from build123d import *

# Parameters (mm, degrees)
SKETCH1_W           = 40
SKETCH1_H           = 30
BOSS_EXTRUDE1_DEPTH = 5
SKETCH2_R           = 1.5
BOSS_EXTRUDE2_DEPTH = 40
SKETCH4_R           = 1.5
BOSS_EXTRUDE4_DEPTH = 5


with BuildPart() as part:
    # Sketch1 → Boss-Extrude1 (new body)
    with BuildSketch(Plane(origin=(0, 0, 0), x_dir=(1, 0, 0), z_dir=(0, 1, 0))):
        with Locations((20, -15)):
            Rectangle(SKETCH1_W, SKETCH1_H)
    extrude(amount=BOSS_EXTRUDE1_DEPTH)

    # Sketch2 → Boss-Extrude2 (add)
    with BuildSketch(Plane.ZY):
        with BuildLine():
            ThreePointArc((8.106694093, 9.054477386), (4.053347046, 13.107824432), (0, 9.054477386))
            Line((0, 9.054477386), (0, 5))
            Line((0, 5), (12.116930909, 5))
            ThreePointArc((12.116930909, 5), (9.279911424, 6.188818307), (8.106633421, 9.032299844))
            ThreePointArc((8.106633421, 9.032299844), (8.106678925, 9.043388574), (8.106694093, 9.054477386))
        make_face()
        with Locations((4.053347046, 9.054477386)):
            Circle(SKETCH2_R, mode=Mode.SUBTRACT)
    extrude(amount=-BOSS_EXTRUDE2_DEPTH)

    # Sketch4 → Boss-Extrude4 (add)
    with BuildSketch(Plane.ZY):
        with BuildLine():
            Line((30, 5), (28.232674565, 29.357717289))
            ThreePointArc((28.232674565, 29.357717289), (24.143809842, 33.243814974), (19.891005174, 29.537843793))
            Line((19.891005174, 29.537843793), (17.041462837, 5))
            Line((17.041462837, 5), (30, 5))
        make_face()
        with Locations((24.053347046, 29.054477386)):
            Circle(SKETCH4_R, mode=Mode.SUBTRACT)
    extrude(amount=-BOSS_EXTRUDE4_DEPTH)


solid = part.part
Model file for the job. Use its own axes, mm. A direction names the side the tool comes from. Coordinates: 2 decimals unless noted, no trailing zeros. Order: outer loops, then holes, each group sorted by start corner. A loop starts at its lowest first (then second) coordinate and runs counter-clockwise, first axis right, second up. Notation, with made-up numbers: (39, 69.25) -> (74, 69.25) arc R27 ccw to (74, 106.25) -> close; hole circle Ø10 at (63.5, 80.25). An arc over 180 degrees is marked (long way). Return JSON: item names as keys, results as strings. Group by question number.
Item 1: Tool access for faces 4 (the flat face through (0, 13, 21)), 5 (the flat face through (5, 16, 23)), 6 (the flat face through (2.465, 17.441, 18.486)): list every direction of +Z, -Z, +X, -X, +Y, -Y with a clear straight run to the whole face (end or side of a thin tool).
Item 2: Saw through at C-C on y = 8.5. Write the cut outline in (x, z), then the cut area to 3 significant figures.
Item 3: Flat gauge pins, fed straight in: P1, Ø2, axis at x = 22, z = 17.5, coming from the +Y side; P2, Ø3.5, axis at y = 29.05, z = 24.05, coming from the +X side; P3, Ø8, axis at x = 9.5, z = 10.5, coming from the +Y side. Where does each tip first touch, or does it go through?
Item 4: Saw through at B-B on z = 3.75. Write the cut outline in (x, y), then the cut area to 3 significant figures.
Item 5: Wall check: line 1 along X through (y, z) = (14, 25.75); line 2 along Y through (x, z) = (15.5, 5.25). Give the ranges that are in metal, low to high. Write a range as [from, to].
Item 6: Saw through at D-D on x = 4. State how many separate pieces and enclosed holes the cut face has, then the cut area to 3 significant figures.
Item 7: Pull direction Z, two halves, no side cores. Call faces 1 (the flat face through (20, 0, 15)), 2 (the cylindrical face through (2.46, 33.24, 24.23)), 3 (the cylindrical face through (19.72, 10.32, 4.86)): pulls with the +Z half, pulls with the -Z half, needs draft (parallel to the pull), parting line crosses it, or undercut.
Values found:
{
 "1": {"face 4": "+Z, -Z, -X, +Y, -Y", "face 5": "+Z, +X, +Y", "face 6": "+X, -X, +Y"},
 "2": {"outline": "(0, 0) -> (40, 0) -> (40, 2.66) -> (0, 2.66) -> close; (0, 5.45) -> (40, 5.45) -> (40, 8.14) -> (0, 8.14) -> close; (0, 17.45) -> (5, 17.45) -> (5, 29.75) -> (0, 29.75) -> close", "area": "276 mm2"},
 "3": {"P1": "stops at y = 5", "P2": "stops at x = 5", "P3": "stops at y = 12.29"},
 "4": {"outline": "(0, 0) -> (40, 0) -> (40, 7.59) -> (0, 7.59) -> close; (0, 10.52) -> (40, 10.52) -> (40, 13.1) -> (0, 13.1) -> close", "area": "406 mm2"},
 "5": {"line 1": "x = [0, 5]", "line 2": "y = [0, 8.15], [9.96, 12.93]"},
 "6": {"separate pieces": "1", "enclosed holes": "2", "area": "483 mm2"},
 "7": {"face 1": "needs draft", "face 2": "parting line crosses it", "face 3": "undercut"}
}
